For this review, take the finished solid that the model builds, in its own axes (mm). Coordinates: 2 decimals unless noted, no trailing zeros. Loops run counter-clockwise (first coordinate to the right, second up) from the corner with the lowest first, then second, coordinate; pieces in that order, holes last.
1. Take a section at A-A, the plane z = -63.5. State the section outline as (x, y) points (3 decimals).
2. To check wall thickness, follow probe 1 along Y at (x, z) = (7.25, 63.5); probe 2 along Z at (x, y) = (2, -21.5); probe 3 along Y at (x, z) = (1.25, -62). State the ranges of each line that lie inside material, in increasing order.
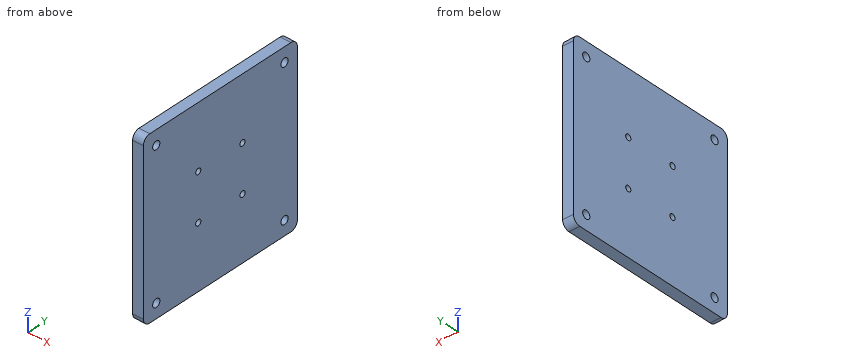
```python
from build123d import *

# Parameters (mm, degrees)
SKETCH1_W               = 152.4
SKETCH1_H               = 152.4
BOSS_EXTRUDE1_DEPTH     = 9.525
F_1_4_20_TAPPED_HOLE1_D = 5.1054
FILLET1_R               = 6.35
F_1_4_CLEARANCE_HOLE1_D = 7.14248


with BuildPart() as part:
    # Sketch1 → Boss-Extrude1 (new body)
    with BuildSketch(Plane(origin=(0, 0, 0), x_dir=(0, 0, -1), z_dir=(1, 0, 0))):
        Rectangle(SKETCH1_W, SKETCH1_H)
    extrude(amount=BOSS_EXTRUDE1_DEPTH)

    # 1/4-20 Tapped Hole1 (through all)
    with Locations(Plane(origin=(9.525, 0, 0), x_dir=(0, 0, -1), z_dir=(1, 0, 0))):
        with Locations((-20.6375, 21.9075), (20.6375, 21.9075), (20.6375, -21.9075), (-20.6375, -21.9075)):
            Hole(F_1_4_20_TAPPED_HOLE1_D / 2)

    # Fillet1
    fillet1_edges = [part.edges().sort_by_distance(p)[0] for p in [
        (4.7625, -76.2, -76.2),
        (4.7625, -76.2, 76.2),
        (4.7625, 76.2, 76.2),
        (4.7625, 76.2, -76.2),
    ]]
    fillet(fillet1_edges, radius=FILLET1_R)

    # 1/4 Clearance Hole1 (through all)
    with Locations(Plane(origin=(9.525, 0, 0), x_dir=(0, 0, -1), z_dir=(1, 0, 0))):
        with Locations((-63.5, 63.5), (63.5, 63.5), (63.5, -63.5), (-63.5, -63.5)):
            Hole(F_1_4_CLEARANCE_HOLE1_D / 2)


solid = part.part
```
Results list:
1. outline: (0, -76.2) - (9.525, -76.2) - (9.525, -67.071) - (0, -67.071) - close; (0, -59.929) - (9.525, -59.929) - (9.525, 59.929) - (0, 59.929) - close; (0, 67.071) - (9.525, 67.071) - (9.525, 76.2) - (0, 76.2) - close
2. probe 1: y = -76.2 to -67.07, -59.93 to 59.93, 67.07 to 76.2
2. probe 2: z = -76.2 to -23.16, -18.12 to 18.12, 23.16 to 76.2
2. probe 3: y = -76.2 to -66.74, -60.26 to 60.26, 66.74 to 76.2
